Job drawing, mm, ordinate dimensions from the low corner. One solid piece. Give positions to 0.01 mm unless a question says otherwise; leave off trailing zeros. Order: outer loops, then holes, each group sorted by start corner. A loop starts at its lowest first (then second) coordinate and runs counter-clockwise, first axis right, second up. Notation, with made-up numbers: M 22,13.25 L 37,13.25 A23 ccw 37,51.25 Z; hole C 67,75.5 d10. An arc over 180 degrees is marked long. One line per question, with ' | ' between items.
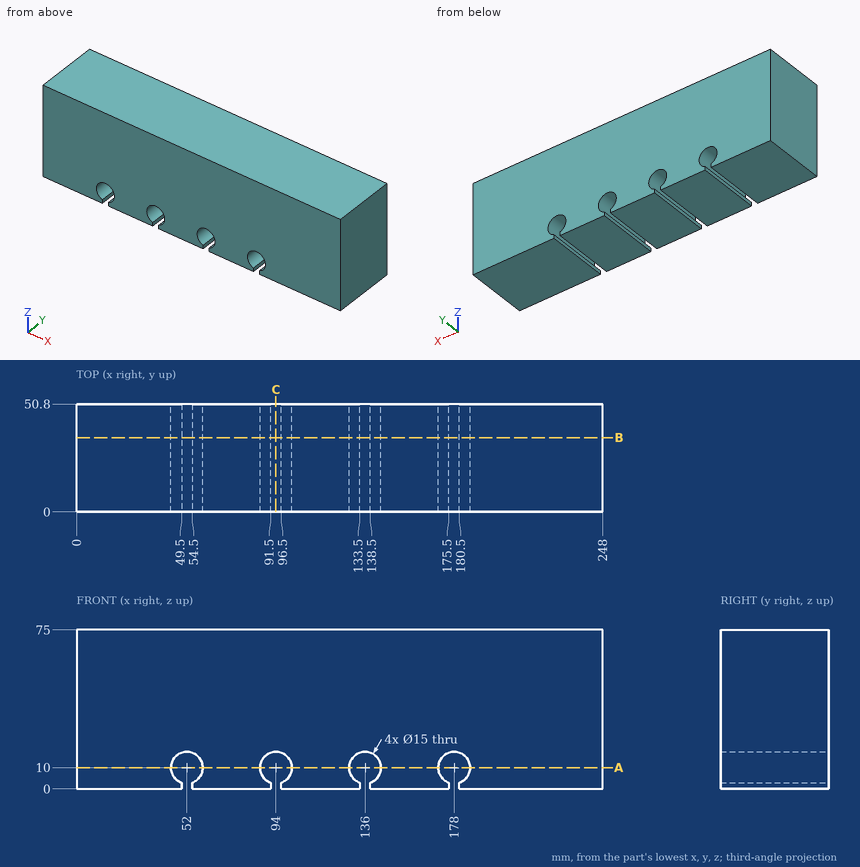
1. Slice it at B-B on y = 35. Give the cut face in (x, z), then the cut area to 3 significant figures.
Worked out:
outline: M 0,0 L 49.5,0 L 49.5,2.93 A7.5 cw long 54.5,2.93 L 54.5,0 L 91.5,0 L 91.5,2.93 A7.5 cw long 96.5,2.93 L 96.5,0 L 133.5,0 L 133.5,2.93 A7.5 cw long 138.5,2.93 L 138.5,0 L 175.5,0 L 175.5,2.93 A7.5 cw long 180.5,2.93 L 180.5,0 L 248,0 L 248,75 L 0,75 Z | area: 17,800 mm2
2. Slice it at C-C on x = 94. Give the cut face in (y, z), then the cut area to 3 significant figures.
Worked out:
outline: M 0,17.5 L 50.8,17.5 L 50.8,75 L 0,75 Z | area: 2,920 mm2
3. Slice it at A-A on z = 10. Give the cut face in (x, y).
Worked out:
outline: M 0,0 L 44.5,0 L 44.5,50.8 L 0,50.8 Z; M 59.5,0 L 86.5,0 L 86.5,50.8 L 59.5,50.8 Z; M 101.5,0 L 128.5,0 L 128.5,50.8 L 101.5,50.8 Z; M 143.5,0 L 170.5,0 L 170.5,50.8 L 143.5,50.8 Z; M 185.5,0 L 248,0 L 248,50.8 L 185.5,50.8 Z
4. Probe L1, parallel to X at y = 20, z = 10; L2, parallel to X at y = 43, z = 15; L3, parallel to Z at x = 99, y = 11. List the from-to ranges inside material, lowest first. Write a range as from..to.
Worked out:
L1: x = 0..44.5, 59.5..86.5, 101.5..128.5, 143.5..170.5, 185.5..248 | L2: x = 0..46.41, 57.59..88.41, 99.59..130.41, 141.59..172.41, 183.59..248 | L3: z = 0..4.41, 15.59..75
5. Drop a flat-ended pin along its axis: pin 1 (9 mm diameter, centred on x = 94, z = 10, fed in from -Y). Give the stop position or say it passes through.
Worked out:
pin 1: passes through
